```python
from build123d import *

# Parameters (mm, degrees)
SKETCH2_R                = 63.5
SKETCH2_R_2              = 42.0000049
BOSS_EXTRUDE1_DEPTH      = 9.449999896
SKETCH27_W               = 4.908836101
SKETCH27_H               = 3.175
CIRPATTERN1_COUNT        = 3
M1_2X0_25_TAPPED_HOLE2_D = 0.95
CIRPATTERN2_COUNT        = 12


with BuildPart() as part:
    # Sketch2 → Boss-Extrude1 (new body)
    with BuildSketch(Plane(origin=(0, 0, 0), x_dir=(1, 0, 0), z_dir=(0, 1, 0))):
        Circle(SKETCH2_R)
        Circle(SKETCH2_R_2, mode=Mode.SUBTRACT)
    extrude(amount=BOSS_EXTRUDE1_DEPTH)

    # Sketch27 → Cut-Revolve1 (revolve, cut)
    with BuildSketch(Plane.XY):
        with Locations((61.04558195, 1.5875)):
            Rectangle(SKETCH27_W, SKETCH27_H)
    revolve(axis=Axis((0, 0, 0), (0, 1, 0)), mode=Mode.SUBTRACT)

    # Sketch33 → CBORE for _8 Binding Head Machine Screw1 (revolve, cut)
    with BuildSketch(Plane(origin=(0, 9.449999896, -50.8), x_dir=(0, 0, 1), z_dir=(1, 0, 0))):
        Polygon((0, 0), (0, 503.000674586), (2.2479, 501.65), (2.2479, 2.667), (4.7625, 2.667), (4.7625, 0), align=None)
    cbore_for_8_binding_head_machine_screw1 = revolve(axis=Axis((0, 15.799999896, -50.8), (0, -1, 0)), mode=Mode.SUBTRACT)

    # CirPattern1: CBORE for _8 Binding Head Machine Screw1 ×3 about axis
    cirpattern1_axis = Axis((0, 0, 0), (0, 1, 0))
    for i in range(1, CIRPATTERN1_COUNT):
        add(cbore_for_8_binding_head_machine_screw1.rotate(cirpattern1_axis, i * 360 / CIRPATTERN1_COUNT), mode=Mode.SUBTRACT)

    # M1.2x0.25 Tapped Hole2 (through all)
    with Locations(Plane(origin=(0, 9.449999896, -44.579871472), x_dir=(0, 0, 1), z_dir=(0, 1, 0))):
        with Locations((0, 0)):
            m1_2x0_25_tapped_hole2 = Hole(M1_2X0_25_TAPPED_HOLE2_D / 2)

    # CirPattern2: M1.2x0.25 Tapped Hole2 ×12 about axis
    cirpattern2_axis = Axis((0, 0, 0), (0, 1, 0))
    for i in range(1, CIRPATTERN2_COUNT):
        add(m1_2x0_25_tapped_hole2.rotate(cirpattern2_axis, i * 360 / CIRPATTERN2_COUNT), mode=Mode.SUBTRACT)


solid = part.part
```
Check sheet for the modelled part. Datum: model origin and axes. Units: mm. A direction names the side the tool comes from. Coordinates: 2 decimals unless noted, no trailing zeros. Write each loop counter-clockwise with the first axis right and the second up, starting at its lowest first coordinate (ties: lowest second). Pieces come first, ordered by that corner, then holes. Notation, with made-up numbers: M 38.25,-25.75 L 76.25,-25.75 A21 ccw 76.25,4.25 Z; hole C 71,62 d11. An arc over 180 degrees is marked long. Write item = value, one per line. Start each with the question number.
1. Sectioned sample at A-A (z = -10.5). Record the cut outline in (x, y) (3 decimals).
2. Tool access check on faces 5 (the cylindrical face through (-46.223, 3.439, 25.107)), 6 (the cylindrical face through (-46.496, 1.61, 35.652)), 7 (the cylindrical face through (42.56, 8.14, 29.94)). Record the directions out of +Z, -Z, +X, -X, +Y, -Y that give a thin tool (end or side, any length) a straight path to the whole face; none if there is none.
3. Sectioned sample at C-C (y = 4.75). State how many separate pieces and enclosed holes the cut face has, then the cut area to 3 significant figures.
4. Thickness scan on probe 1 along X at (y, z) = (8.2, -50.8); probe 2 along Y at (x, z) = (-17.5, -57.5) (3 decimals); probe 3 along X at (y, z) = (1, -8). Record the ranges inside material, lowest first.
5. Sectioned sample at B-B (x = -31.5). Record the cut outline in (y, z) (3 decimals), then the cut area to 3 significant figures.
6. Mould release check, pull along Z, two halves, no side actions. Record for faces 1 (the cylindrical face through (-13.77, 6.27, 61.99)), 2 (the flat face through (-46, 6.783, 24)), 3 (the cylindrical face through (41.765, 3.439, 25.107)), 4 (the flat face through (-56, 3.175, 19)): pulls with the +Z half, pulls with the -Z half, needs draft (parallel to the pull), parting line crosses it, or undercut.
7. Go/stop test with flat-tipped pins: pin 1 (12.5 mm diameter, centred on x = 43.99, z = 25.4, fed in from +Y); pin 2 (7.5 mm diameter, centred on x = -43.99, z = 25.4, fed in from +Y); pin 3 (1.5 mm diameter, centred on y = 5.5, z = 34.5, fed in from -X). Record where each tip stops, or that it passes through.
The answers:
q1.outline = M -62.626,3.175 L -57.643,3.175 L -57.643,0 L -40.666,0 L -40.666,9.45 L -62.626,9.45 Z; M 40.666,0 L 57.643,0 L 57.643,3.175 L 62.626,3.175 L 62.626,9.45 L 40.666,9.45 Z
q2.face_5 = +Y, -Y
q2.face_6 = -Y
q2.face_7 = +Y
q3.separate_pieces = 1
q3.enclosed_holes = 16
q3.area = 7,070 mm²
q4.probe_1 = -38.1 to -4.76, 4.76 to 38.1
q4.probe_2 = 3.175 to 9.45
q4.probe_3 = -58.04 to -41.23, 41.23 to 58.04
q5.outline = M 0,-49.403 L 3.175,-49.403 L 3.175,-55.136 L 9.45,-55.136 L 9.45,-27.78 L 0,-27.78 Z; M 0,27.78 L 9.45,27.78 L 9.45,55.136 L 3.175,55.136 L 3.175,49.403 L 0,49.403 Z
q5.area = 481 mm²
q6.face_1 = parting line crosses it
q6.face_2 = undercut
q6.face_3 = undercut
q6.face_4 = needs draft
q7.pin_1 = 9.45
q7.pin_2 = 6.78
q7.pin_3 = -53.79
